The listing builds one solid part. Answer for the finished solid, in the listing's coordinates (mm). Round coordinates to 2 decimals unless told otherwise and drop trailing zeros. Write each loop counter-clockwise with the first axis right and the second up, starting at its lowest first coordinate (ties: lowest second). Pieces come first, ordered by that corner, then holes. Notation, with made-up numbers: (59, 41.25) - (70, 41.25) arc R31 cw to (70, 78.25) - close; hole circle Ø6 at (47, -26). An arc over 180 degrees is marked (long way). Answer as CSV lines item,"result". Start each with the question number.
Item 1: A cutting plane is placed at A-A on y = 18.5. Determine the outline of the cut face in (x, z), and give its area (3 significant figures).
Item 2: A cutting plane is placed at C-C on x = 25. Determine the outline of the cut face in (y, z).
Item 3: A flat-ended cylindrical pin translates along its axis: pin 1 (6 mm diameter, centred on y = 35.5, z = -17, fed in from -X). Find the tip coordinate at first contact, or state that the pin passes through.
Item 4: A cutting plane is placed at B-B on z = -10. Determine the outline of the cut face in (x, y).
Item 5: Straight lines are drawn through the part: line 1 along X through (y, z) = (9, -26); line 2 along X through (y, z) = (33.5, -24.5). For each, find the intervals that lie inside material, in ascending order. Write a range as [from, to].
Solid Edge part; units mm, degrees
sketch "Sketch1" plane through (0, 0, 0) normal (0, -1, 0) x (1, 0, 0)
  line L0 (0, -32) -> (250, -32)
  line L1 (250, -32) -> (250, 0)
  line L2 (250, 0) -> (0, 0)
  line L3 (0, 0) -> (0, -32)
extrude "Protrusion1" add sketch "Sketch1" against normal blind 40
sketch "Sketch2" plane through (125, 0, -16) normal (0, -1, 0) x (1, 0, 0)
  line L0 (-70, 16) -> (-125, 5.8064)
  line L1 (-125, 5.8064) -> (-125, 16)
  line L2 (-125, 16) -> (-70, 16)
extrude "ExtrudedCutout_1" cut sketch "Sketch2" against normal blind 40
fillet "Round_1" radius 20 2 edges at (0, 20, -10.1936) (55, 20, 0)
Geometry says:
1,outline,"(0, -32) - (250, -32) - (250, 0) - (56.84, 0) arc R20 ccw to (53.19, -0.33) - (16.36, -7.16) arc R20 ccw to (0, -26.83) - close"
1,area,"7,660 mm^2"
2,outline,"(0, -32) - (40, -32) - (40, -5.56) - (0, -5.56) - close"
3,pin 1,"stops at x = 1.2"
4,outline,"(9.19, 0) - (250, 0) - (250, 40) - (9.19, 40) - close"
5,line 1,"x = [0.02, 250]"
5,line 2,"x = [0.14, 250]"
